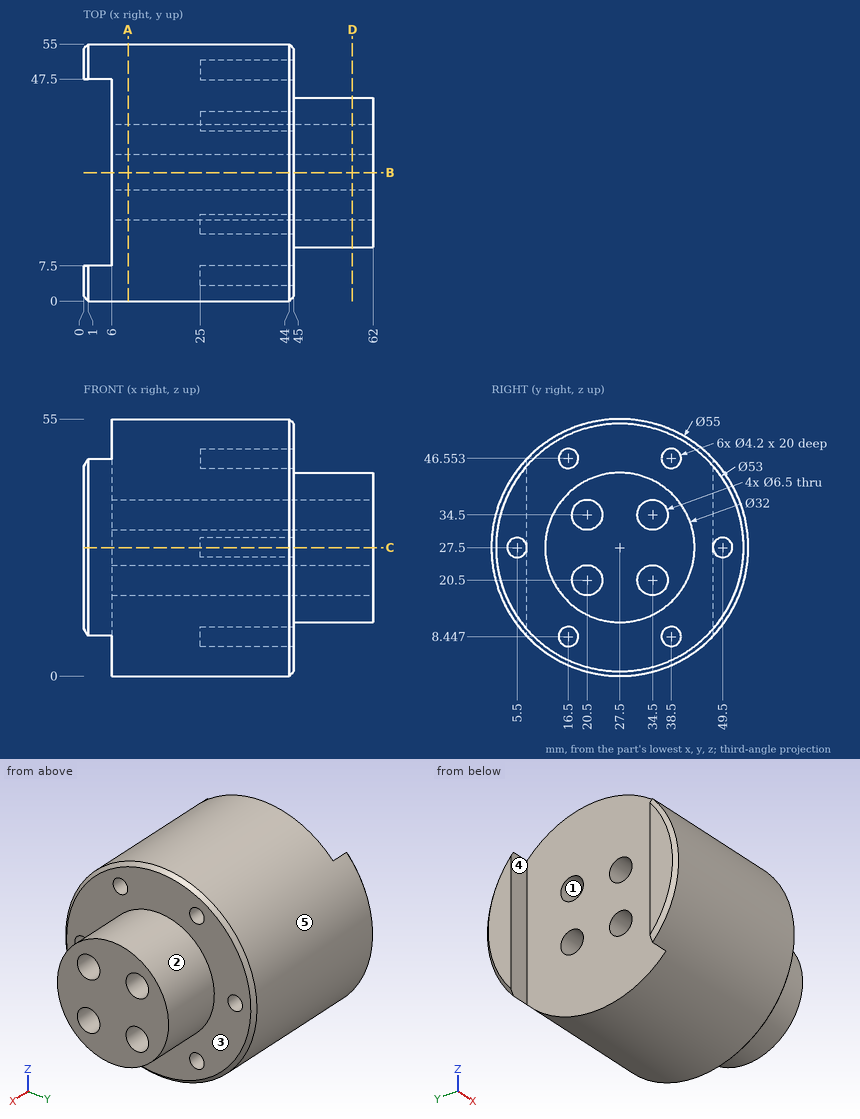
Answer from the drawing. Dimensions are ordinates in mm from the lowest x, y and z of the part. A direction names the side the tool comes from. Give positions to 0.01 mm unless a question says otherwise; leave off trailing zeros. Write each loop counter-clockwise with the first axis right and the second up, starting at its lowest first coordinate (ties: lowest second). Pieces come first, ordered by that corner, then holes. Notation, with made-up numbers: (39.25, 34.25) - (64.25, 34.25) arc R26 ccw to (64.25, 59.25) - close; hole circle Ø6 at (7, -4). An arc over 180 degrees is marked (long way). Answer in a Markdown table with one row per item. Add a question column.
Item 1: Section A-A, the plane x = 9.5 is taken. Write down the section's boundary in (y, z), and give its area (3 significant figures).
Item 2: Determine the mould class of the marked faces 1, 2 and 3 for opening direction Z: pulls with the +Z half, pulls with the -Z half, needs draft (parallel to the pull), parting line crosses it, or undercut.
Item 3: Section D-D, the plane x = 57.5 is taken. Write down the section's boundary in (y, z).
Item 4: Section C-C, the plane z = 27.5 is taken. Write down the section's boundary in (x, y).
Item 5: A tool of negligible diameter and unlimited length cuts with its end or side. For the marked faces 4 and 5, from which of +Z, -Z, +X, -X, +Y, -Y can it reach the whole face along a straight path? Write none if from no direction.
Item 6: Flat-ended cylindrical pins translate along their axes: P1, Ø3.5, axis at y = 38.5, z = 8.45, coming from the -X side; P2, Ø2, axis at x = 38.5, y = 39, coming from the -Z side; P3, Ø4, axis at y = 26, z = 9, coming from the +X side; P4, Ø4, axis at y = 34.5, z = 34.5, coming from the +X side. Find the tip coordinate at first contact, or state that the pin passes through.
Item 7: Find the intervals of material crossed by L1, parallel to Y at x = 31, z = 34; L2, parallel to Y at x = 40, z = 28 (1 decimal); L3, parallel to X at y = 11.5, z = 32.5, in increasing order.
Item 8: Section B-B, the plane y = 27.5 is taken. Write down the section's boundary in (x, z).
Recorded:
| question | item | result |
|---|---|---|
| 1 | outline | circle Ø55 at (27.5, 27.5); hole circle Ø6.5 at (20.5, 20.5); hole circle Ø6.5 at (20.5, 34.5); hole circle Ø6.5 at (34.5, 20.5); hole circle Ø6.5 at (34.5, 34.5) |
| 1 | area | 2,240 mm2 |
| 2 | face 1 | undercut |
| 2 | face 2 | parting line crosses it |
| 2 | face 3 | needs draft |
| 3 | outline | circle Ø32 at (27.5, 27.5); hole circle Ø6.5 at (20.5, 20.5); hole circle Ø6.5 at (20.5, 34.5); hole circle Ø6.5 at (34.5, 20.5); hole circle Ø6.5 at (34.5, 34.5) |
| 4 | outline | (0, 1) - (1, 0) - (44, 0) - (45, 1) - (45, 3.4) - (25, 3.4) - (25, 7.6) - (45, 7.6) - (45, 11.5) - (62, 11.5) - (62, 43.5) - (45, 43.5) - (45, 47.4) - (25, 47.4) - (25, 51.6) - (45, 51.6) - (45, 54) - (44, 55) - (1, 55) - (0, 54) - (0, 47.5) - (6, 47.5) - (6, 7.5) - (0, 7.5) - close |
| 5 | face 4 | +Z, -Z, -X |
| 5 | face 5 | +X, -X |
| 6 | P1 | stops at x = 6 |
| 6 | P2 | stops at z = 2.08 |
| 6 | P3 | stops at x = 45 |
| 6 | P4 | passes through |
| 7 | L1 | y = 0.78 to 17.29, 23.71 to 31.29, 37.71 to 54.22 |
| 7 | L2 | y = 0 to 3.5, 7.5 to 47.5, 51.5 to 55 |
| 7 | L3 | x = 6 to 45 |
| 8 | outline | (6, 0) - (44, 0) - (45, 1) - (45, 11.5) - (62, 11.5) - (62, 43.5) - (45, 43.5) - (45, 54) - (44, 55) - (6, 55) - close |
